Here's how the part is built. I have some questions about the finished solid (model axes, mm). Face numbers are marked on the shaded views. A direction names the side the tool comes from. Give positions to 0.01 mm unless a question says otherwise; leave off trailing zeros. Write each loop counter-clockwise with the first axis right and the second up, starting at its lowest first coordinate (ties: lowest second). Pieces come first, ordered by that corner, then holes. Notation, with made-up numbers: (25.5, 51) - (77.5, 51) arc R25 ccw to (77.5, 63) - close; hole circle Ø7 at (-21, 28). An arc over 180 degrees is marked (long way). Use a Markdown table: item, result.
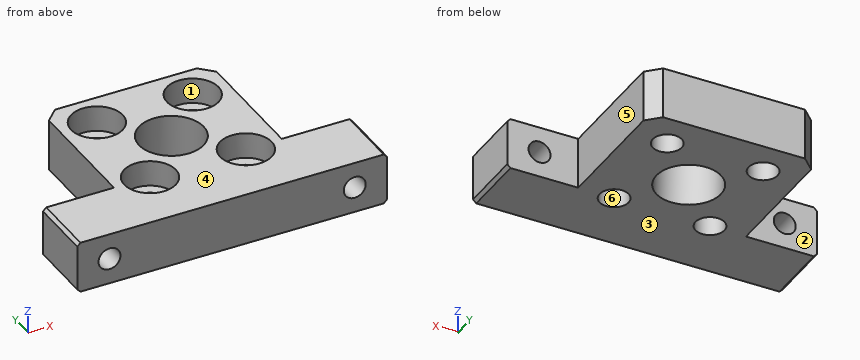
```python
from build123d import *

# Parameters (mm, degrees)
SKETCH1_R           = 2.25
SKETCH1_R_2         = 5
BOSS_EXTRUDE1_DEPTH = 8
SKETCH2_R           = 4
CUT_EXTRUDE1_DEPTH  = 4
SKETCH3_R           = 1.701572747
CUT_EXTRUDE2_DEPTH  = 32
CHAMFER1_SIZE       = 2
CHAMFER2_SIZE       = 0.5


with BuildPart() as part:
    # Sketch1 → Boss-Extrude1 (new body)
    with BuildSketch(Plane.XY):
        Polygon((16.978142077, -11.01947541), (27.978142077, -11.01947541), (27.978142077, -21.01947541), (-20.021857923, -21.01947541), (-20.021857923, -11.01947541), (-9.021857923, -11.01947541), (-9.021857923, 9.98052459), (16.978142077, 9.98052459), align=None)
        with Locations((-3.437114754, -11.01947541)):
            Circle(SKETCH1_R, mode=Mode.SUBTRACT)
        with Locations((11.416131148, -11.01947541)):
            Circle(SKETCH1_R, mode=Mode.SUBTRACT)
        with Locations((-3.437114754, 4.48052459)):
            Circle(SKETCH1_R, mode=Mode.SUBTRACT)
        with Locations((11.416131148, 4.48052459)):
            Circle(SKETCH1_R, mode=Mode.SUBTRACT)
        with Locations((3.978142077, -3.26947541)):
            Circle(SKETCH1_R_2, mode=Mode.SUBTRACT)
    extrude(amount=BOSS_EXTRUDE1_DEPTH)

    # Sketch2 → Cut-Extrude1 (cut)
    with BuildSketch(Plane.XY.offset(8)):
        with Locations((-3.437114754, 4.48052459)):
            Circle(SKETCH2_R)
        with Locations((11.416131148, 4.48052459)):
            Circle(SKETCH2_R)
        with Locations((-3.437114754, -11.01947541)):
            Circle(SKETCH2_R)
        with Locations((11.416131148, -11.01947541)):
            Circle(SKETCH2_R)
    extrude(amount=-CUT_EXTRUDE1_DEPTH, mode=Mode.SUBTRACT)

    # Sketch3 → Cut-Extrude2 (cut, through all)
    with BuildSketch(Plane(origin=(0, 9.98052459, 0), x_dir=(1, 0, 0), z_dir=(0, 1, 0))):
        with Locations((-15.021857923, -4)):
            Circle(SKETCH3_R)
        with Locations((22.978142077, -4)):
            Circle(SKETCH3_R)
    extrude(amount=-CUT_EXTRUDE2_DEPTH, mode=Mode.SUBTRACT)

    # Chamfer1
    chamfer1_edges = [part.edges().sort_by_distance(p)[0] for p in [
        (-9.021857923, 9.98052459, 4),
        (16.978142077, 9.98052459, 4),
    ]]
    chamfer(chamfer1_edges, length=CHAMFER1_SIZE)

    # Chamfer2
    chamfer2_edges = [part.edges().sort_by_distance(p)[0] for p in [
        (-20.021857923, -16.01947541, 8),
        (27.978142077, -16.01947541, 8),
        (27.978142077, -16.01947541, 0),
        (-20.021857923, -16.01947541, 0),
    ]]
    chamfer(chamfer2_edges, length=CHAMFER2_SIZE)


solid = part.part
```
Item 1: If we section it at B-B, the plane y = -1: Write out the boundary of the cut face in (x, z).
Values:
| item | result |
|---|---|
| outline | (-9.02, 0) - (-0.48, 0) - (-0.48, 8) - (-9.02, 8) - close; (8.43, 0) - (16.98, 0) - (16.98, 8) - (8.43, 8) - close |
Item 2: If we section it at C-C, the plane x = 12: Write out the boundary of the cut face in (y, z).
Values:
| item | result |
|---|---|
| outline | (-21.02, 0) - (-13.19, 0) - (-13.19, 4) - (-14.98, 4) - (-14.98, 8) - (-21.02, 8) - close; (-8.85, 0) - (2.31, 0) - (2.31, 4) - (0.52, 4) - (0.52, 8) - (-7.06, 8) - (-7.06, 4) - (-8.85, 4) - close; (6.65, 0) - (9.98, 0) - (9.98, 8) - (8.44, 8) - (8.44, 4) - (6.65, 4) - close |
Item 3: For the marked faces 1, 2 and 3, which set-ups out of +Z, -Z, +X, -X, +Y, -Y let a thin tool reach every point of the face, with its end or its side?
Values:
| item | result |
|---|---|
| face 1 | +Z |
| face 2 | +Z, -Z, -X, +Y |
| face 3 | -Z, +X, -X, +Y, -Y |
Item 4: Thinking about a two-plate mould opening in X: for the marked faces 4, 5 and 6, which applies, +X half, -X half, draft (parallel to the pull), parting line (faces both ways), or undercut?
Values:
| item | result |
|---|---|
| face 4 | draft |
| face 5 | +X half |
| face 6 | undercut |
Item 5: If we section it at D-D, the plane y = -12: Write out the boundary of the cut face in (x, z), plus the area to 3 significant figures.
Values:
| item | result |
|---|---|
| outline | (-20.02, 0.5) - (-19.52, 0) - (-5.46, 0) - (-5.46, 4) - (-7.32, 4) - (-7.32, 8) - (-19.52, 8) - (-20.02, 7.5) - close; (-1.41, 0) - (9.39, 0) - (9.39, 4) - (7.54, 4) - (7.54, 8) - (0.44, 8) - (0.44, 4) - (-1.41, 4) - close; (13.44, 0) - (27.48, 0) - (27.98, 0.5) - (27.98, 7.5) - (27.48, 8) - (15.29, 8) - (15.29, 4) - (13.44, 4) - close; hole circle Ø3.4 at (-15.02, 4); hole circle Ø3.4 at (22.98, 4) |
| area | 271 mm2 |
Item 6: If we section it at A-A, the plane z = 3: Write out the boundary of the cut face in (x, y).
Values:
| item | result |
|---|---|
| outline | (-20.02, -21.02) - (-16.4, -21.02) - (-16.4, -11.02) - (-20.02, -11.02) - close; (-13.65, -21.02) - (21.6, -21.02) - (21.6, -11.02) - (16.98, -11.02) - (16.98, 7.98) - (14.98, 9.98) - (-7.02, 9.98) - (-9.02, 7.98) - (-9.02, -11.02) - (-13.65, -11.02) - close; (24.35, -21.02) - (27.98, -21.02) - (27.98, -11.02) - (24.35, -11.02) - close; hole circle Ø4.5 at (-3.44, -11.02); hole circle Ø4.5 at (-3.44, 4.48); hole circle Ø10 at (3.98, -3.27); hole circle Ø4.5 at (11.42, -11.02); hole circle Ø4.5 at (11.42, 4.48) |
Item 7: I need wall thicknesses on line 1 along X through (y, z) = (-3, 5.75); line 2 along Y through (x, z) = (-3.5, 3); line 3 along Y through (x, z) = (10.5, 4.5). Which ranges of each line are inside material? Lowest first, please. Write a range as [from, to].
Values:
| item | result |
|---|---|
| line 1 | x = [-9.02, -1.01], [8.97, 16.98] |
| line 2 | y = [-21.02, -13.27], [-8.77, 2.23], [6.73, 9.98] |
| line 3 | y = [-21.02, -14.91], [-7.13, 0.59], [8.37, 9.98] |
Item 8: Will these pins go through, and if not, where does the flat tip stop? pin 1 Ø2.5 at (x, y) = (-3, 3) entering from +Z; pin 2 Ø9 at (x, y) = (-3, -11) entering from +Z; pin 3 Ø4 at (x, z) = (20.5, 5) entering from +Y; pin 4 Ø2.5 at (x, z) = (22.98, 4) entering from +Y.
Values:
| item | result |
|---|---|
| pin 1 | stops at z = 4 |
| pin 2 | stops at z = 8 |
| pin 3 | stops at y = -11.02 |
| pin 4 | passes through |
